Here's the drawing with two shaded views (mm, measured from the low corner). I have some questions. Give positions to 0.01 mm unless a question says otherwise; leave off trailing zeros. Loops run counter-clockwise (first coordinate to the right, second up) from the corner with the lowest first, then second, coordinate; pieces in that order, holes last. Notation, with made-up numbers: (-22, -29) - (18, -29) arc R6 cw to (18, -18) - close; hole circle Ø3 at (-30, -9). An arc over 180 degrees is marked (long way). Write each question's results on one line, items separated by ' | '. Start each with the question number.
1) I want a section at C-C, the plane x = 3. Count the separate pieces of the cut face and the enclosed holes in it, and give its area (3 significant figures).
2) I want a section at B-B, the plane y = 148.5. Write out the boundary of the cut face in (x, z).
3) If I drill on probe 1 along Y at (x, z) = (3.85, 35); probe 2 along Z at (x, y) = (4.2, 150); probe 3 along Z at (x, y) = (5.1, 253.5), over which ranges is the centre line in solid material (lowest first)? Write a range as [from, to].
4) I'm going to push flat-ended pins straight in: pin 1 (3 mm diameter, centred on x = 3, z = 26.5, fed in from -Y); pin 2 (3 mm diameter, centred on x = 2.5, y = 3.5, fed in from -Z); pin 3 (3 mm diameter, centred on x = 4.5, y = 45.5, fed in from +Z); pin 4 (25 mm diameter, centred on y = 150, z = 31, fed in from -X). Where does each tip first touch, or does it pass through?
5) I want a section at A-A, the plane z = 31. Write out the boundary of the cut face in (x, y), and give its area (3 significant figures).
6) I want a section at D-D, the plane y = 68.5. Write out the boundary of the cut face in (x, z).
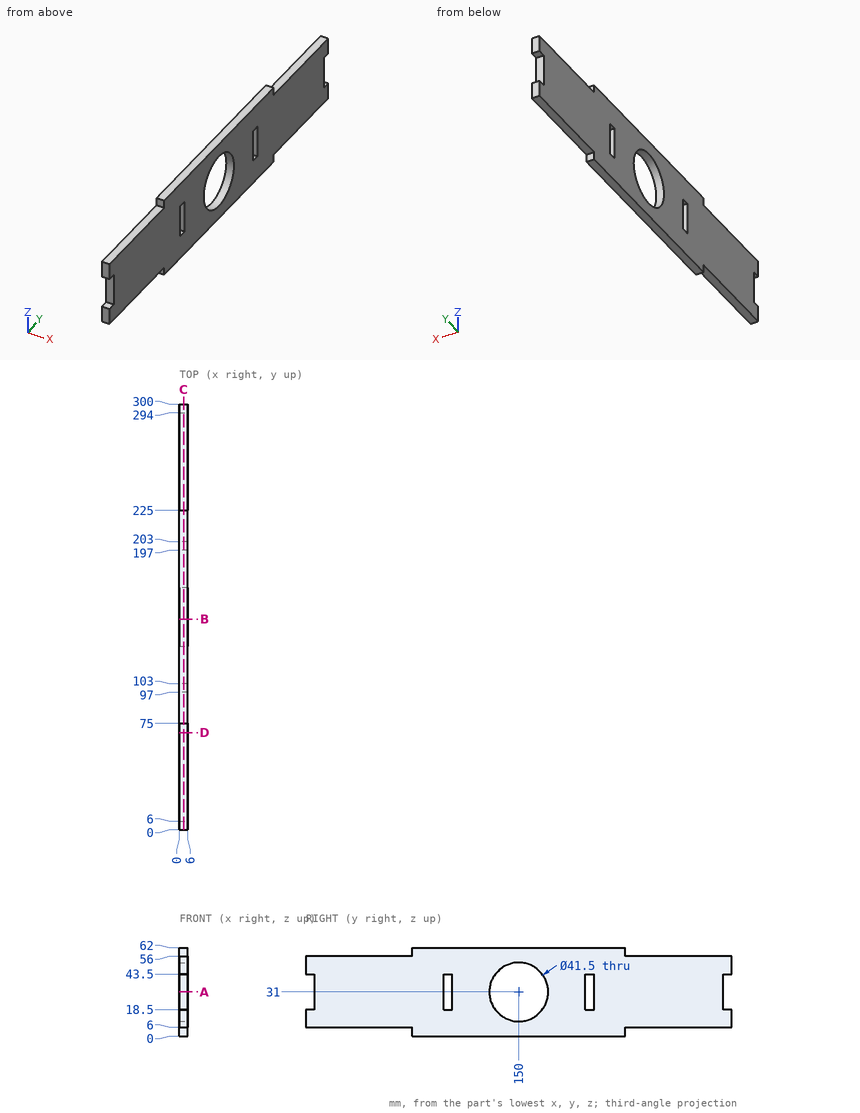
Answers:
1) separate pieces: 1 | enclosed holes: 3 | area: 14,800 mm2
2) outline: (0, 0) - (6, 0) - (6, 10.3) - (0, 10.3) - close; (0, 51.7) - (6, 51.7) - (6, 62) - (0, 62) - close
3) probe 1: y = [6, 97], [103, 129.64], [170.36, 197], [203, 294] | probe 2: z = [0, 10.25], [51.75, 62] | probe 3: z = [6, 56]
4) pin 1: stops at y = 6 | pin 2: stops at z = 6 | pin 3: stops at z = 56 | pin 4: passes through
5) outline: (0, 6) - (6, 6) - (6, 97) - (0, 97) - close; (0, 103) - (6, 103) - (6, 129.25) - (0, 129.25) - close; (0, 170.75) - (6, 170.75) - (6, 197) - (0, 197) - close; (0, 203) - (6, 203) - (6, 294) - (0, 294) - close | area: 1,410 mm2
6) outline: (0, 6) - (6, 6) - (6, 56) - (0, 56) - close
